Source: CAD feature listing. Evaluate the final solid. Frame: model axes, mm. A direction names the side the tool comes from. Coordinates: 2 decimals unless noted, no trailing zeros. Order: outer loops, then holes, each group sorted by start corner. A loop starts at its lowest first (then second) coordinate and runs counter-clockwise, first axis right, second up.
```python
from build123d import *

# Parameters (mm, degrees)
F0_W     = 114.3
F0_H     = 165.1
F1_DEPTH = 4.3434
F3_W     = 12.7
F3_H     = 4.3434
F4_DEPTH = 4.3444
F5_W     = 12.7
F5_H     = 4.3434
F6_DEPTH = 4.3444


with BuildPart() as f1:
    # F0 (on Top) → F1 (new body)
    with BuildSketch(Plane.XY):
        with Locations((0.885719, 52.846001)):
            Rectangle(F0_W, F0_H)
    extrude(amount=F1_DEPTH)

    # F3 (on Top) → F4 (cut, through all)
    with BuildSketch(Plane.XY):
        with Locations((1.166433, -27.752964)):
            Rectangle(F3_W, F3_H)
    extrude(amount=F4_DEPTH, mode=Mode.SUBTRACT)

    # F5 (on Top) → F6 (cut, through all)
    with BuildSketch(Plane.XY):
        with Locations((0.897519, 133.60057)):
            Rectangle(F5_W, F5_H)
    extrude(amount=F6_DEPTH, mode=Mode.SUBTRACT)


solid = f1.part
```
Q1. Section query A-A on x = 2. Output: boundary loops of the cut face in (y, z), plus the area to 3 significant figures.
Solutions:
outline: (-25.58, 0) - (131.43, 0) - (131.43, 4.34) - (-25.58, 4.34) - close
area: 682 mm2
Q2. Pin query (flat end, axial travel): P1, Ø3, axis at x = -18.5, y = 54.5, coming from the -Z side; P2, Ø2, axis at x = 1.5, z = 3, coming from the -Y side; P3, Ø2, axis at x = -0.5, z = 1.5, coming from the +Y side. Return the tip coordinate at first contact, or that it passes through.
Solutions:
P1: stops at z = 0
P2: stops at y = -25.58
P3: stops at y = 131.43
Q3. Set-up query: faces 1 (the flat face through (1, -25.581, 2)), 2 (the flat face through (1, 131.429, 2)), 3 (the flat face through (0, 54, 0)). Return all of +Z, -Z, +X, -X, +Y, -Y with unobstructed straight access to the full face (end or side cutting, diameter ignored); none if empty.
Solutions:
face 1: +Z, -Z, -Y
face 2: +Z, -Z, +Y
face 3: -Z, +X, -X, +Y, -Y
Q4. Material intervals for line 1 along Y through (x, z) = (1, 1.4), sorted ascending.
Solutions:
line 1: y = -25.58 to 131.43
